Can you work these out from the model? Positions are in its coordinate system, mm. A direction names the side the tool comes from. Give positions to 0.01 mm unless a question says otherwise; leave off trailing zeros. Loops run counter-clockwise (first coordinate to the right, second up) from the corner with the lowest first, then second, coordinate; pieces in that order, holes last. Notation, with made-up numbers: (1, 42.25) -> (30, 42.25) arc R12 cw to (30, 54.25) -> close; hole circle Ø11 at (1, -39.5). An arc over 180 degrees is marked (long way). Return JSON: item names as keys, results as strings. Group by question number.
Q1. Which directions (+Z, -Z, +X, -X, +Y, -Y) give clear straight access to the entire face, cutting with the end or side of a thin tool? Please do faces 5 (the flat face through (7, 76, -0.75)), 6 (the flat face through (0.75, 76, 7)), 7 (the flat face through (-7, 76, -0.75)), 8 (the flat face through (3, 146.2, 3)), 9 (the flat face through (-0.75, 76, 7)).
Q2. I need wall thicknesses on line 1 along Y through (x, z) = (-9, 5.5); line 2 along X through (y, z) = (117, 9). Which ranges of each line are inside material? Lowest first, please. Write a range as [from, to].
Q3. Suppose I cut it at B-B, the plane x = -7.5. Please give me the cut outline in (y, z).
Q4. Suppose I cut it at A-A, the plane y = 120. Please give me the cut outline in (x, z), and give its area (4 significant figures).
Q5. Thinking about a two-plate mould opening in Y: for faces 1 (the flat face through (0.75, 76, -7)), 2 (the flat face through (-7, 76, 0.75)), 3 (the flat face through (0, 149.2, 0)), 4 (the cylindrical face through (15.5, 147.68, 4.88)), which applies, pulls with the +Y half, pulls with the -Y half, needs draft (parallel to the pull), parting line crosses it, or undercut?
Q6. Will these pins go through, and if not, where does the flat tip stop? pin 1 (10 mm diameter, centred on x = 9, y = 44.5, fed in from +Z); pin 2 (10 mm diameter, centred on x = -5.5, y = 81, fed in from +Z); pin 3 (10 mm diameter, centred on x = -5, z = 3.5, fed in from -Y); pin 4 (0.8 mm diameter, centred on x = 0, y = 88, fed in from -Z).
Autodesk Inventor part; units mm, degrees
ref_plane "YZ Plane" through (0, 0, 0) normal (1, 0, 0) x (0, 1, 0)
ref_plane "XZ Plane" through (0, 0, 0) normal (0, 1, 0) x (-1, 0, 0)
sketch "Sketch1" plane through (0, 0, 0) normal (0, 1, 0) x (-1, 0, 0)
  circle A0 centre (0, 0) radius 14
  dimension "d0" = 28
extrude "Extrusion1" add sketch "Sketch1" along normal blind 8.2
sketch "Sketch2" plane through (0, 8.2, 0) normal (0, 1, 0) x (1, 0, 0)
  line L0 (-13.5, -0.75) -> (-13.5, 0.75)
  line L1 (13.5, 0.75) -> (13.5, -0.75)
  line L2 (13.5, -0.75) -> (-13.5, 0.75) construction
  line L3 (-13.5, -0.75) -> (13.5, 0.75) construction
  line L4 (0.75, -13.5) -> (-0.75, -13.5)
  line L5 (-0.75, 13.5) -> (0.75, 13.5)
  line L6 (0.75, -13.5) -> (-0.75, 13.5) construction
  line L7 (-0.75, -13.5) -> (0.75, 13.5) construction
  line L8 (-0.75, -13.5) -> (-0.75, -0.75)
  line L9 (-0.75, 0.75) -> (-0.75, 13.5)
  line L10 (-13.5, 0.75) -> (-0.75, 0.75)
  line L11 (13.5, -0.75) -> (0.75, -0.75)
  line L12 (-0.75, -0.75) -> (-13.5, -0.75)
  line L13 (0.75, 13.5) -> (0.75, 0.75)
  line L14 (0.75, -0.75) -> (0.75, -13.5)
  line L15 (0.75, 0.75) -> (13.5, 0.75)
  point P0 (0, 0)
  dimension "d3" = 1.5
  dimension "d4" = 27
  dimension "d5" = 27
extrude "Extrusion2" add sketch "Sketch2" along normal blind 138
sketch "Sketch3" plane through (0, 146.2, 0) normal (0, 1, 0) x (1, 0, 0)
  circle A0 centre (0, 0) radius 16.25
  dimension "d8" = 32.5
extrude "Extrusion3" add sketch "Sketch3" along normal blind 3
equation "\"d5\" = d4"
equation "\"d18\" = d17"
properties part number "CH_01_0007_piston"
Ans:
{
 "1": {"face 5": "-Z, +X", "face 6": "+Z, +X", "face 7": "-Z, -X", "face 8": "none", "face 9": "+Z, -X"},
 "2": {"line 1": "y = [0, 8.2], [146.2, 149.2]", "line 2": "x = [-0.75, 0.75]"},
 "3": {"outline": "(0, -11.82) -> (8.2, -11.82) -> (8.2, -0.75) -> (146.2, -0.75) -> (146.2, -14.42) -> (149.2, -14.42) -> (149.2, 14.42) -> (146.2, 14.42) -> (146.2, 0.75) -> (8.2, 0.75) -> (8.2, 11.82) -> (0, 11.82) -> close"},
 "4": {"outline": "(-13.5, -0.75) -> (-0.75, -0.75) -> (-0.75, -13.5) -> (0.75, -13.5) -> (0.75, -0.75) -> (13.5, -0.75) -> (13.5, 0.75) -> (0.75, 0.75) -> (0.75, 13.5) -> (-0.75, 13.5) -> (-0.75, 0.75) -> (-13.5, 0.75) -> close", "area": "78.75 mm^2"},
 "5": {"face 1": "undercut", "face 2": "undercut", "face 3": "pulls with the +Y half", "face 4": "needs draft"},
 "6": {"pin 1": "stops at z = 0.75", "pin 2": "stops at z = 13.5", "pin 3": "stops at y = 0", "pin 4": "stops at z = -13.5"}
}
